Read the model definition and answer for the solid it produces. Units are mm, in the model's axes. Face numbers are marked on the shaded views. A direction names the side the tool comes from. Coordinates: 2 decimals unless noted, no trailing zeros. Order: outer loops, then holes, each group sorted by start corner. A loop starts at its lowest first (then second) coordinate and runs counter-clockwise, first axis right, second up. Notation, with made-up numbers: M 71.5,38 L 120.5,38 A16 cw 120.5,56 Z; hole C -2,-26 d6. An arc over 180 degrees is marked long. Use a Markdown table: item, result. Add a question column.
1) Find the intervals of material crossed by probe 1 along X at (y, z) = (49, 1.75); probe 2 along Y at (x, z) = (2.5, 2); probe 3 along X at (y, z) = (73, 3), in increasing order. Write a range as [from, to].
2) Each of these flat-tipped pins is pushed along its axis until it touches: pin 1 Ø7.5 at (x, y) = (58, 50) entering from -Z; pin 2 Ø1 at (y, z) = (57, 1) entering from -X; pin 3 Ø1.2 at (x, z) = (1, 0.5) entering from -Y; pin 4 Ø2.5 at (x, y) = (-59.98, 54.01) entering from +Z. Where does it stop, or does it pass through?
3) Find section A-A on z = 3.75. Write down the section's boundary in (x, y), plus the area to 3 significant figures.
4) The mould has two halves that part along X. Classify the marked faces 4, 5, 6 and 7: released by +X, released by -X, zero draft, split by the parting line, or undercut.
5) For the marked faces 1, 2 and 3, determine the directions among +Z, -Z, +X, -X, +Y, -Y from which every point of the face is accessible in a straight line to the end or side of a thin tool.
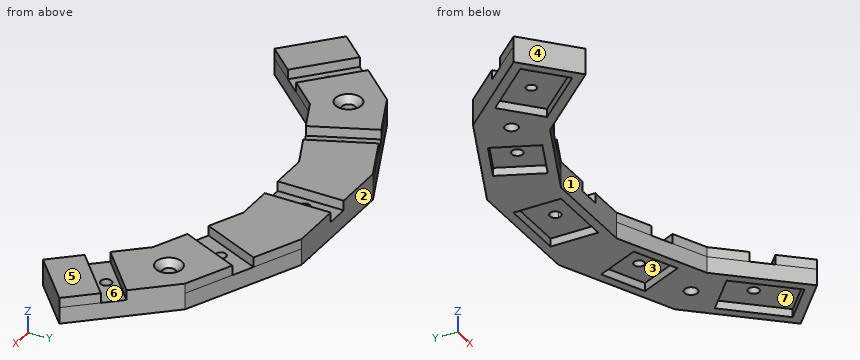
from build123d import *

# Parameters (mm, degrees)
F1_DEPTH       = 5
F3_DEPTH       = 3
F6_D           = 4
F6_CSINK_D     = 8
F6_CSINK_ANGLE = 90
F4_R           = 1.5456356791
F4_R_2         = 1.6934971507
F4_R_3         = 1.5922062155
F4_R_4         = 1.6882702818
F7_DEPTH       = 11.1
F9_DEPTH       = 2.5
F10_R          = 1.4984626167
F11_DEPTH      = 1
F12_R          = 1.6745754143
F13_DEPTH      = 1
F14_W          = 7
F14_H          = 20.1999992132
F14_R          = 1.6202134685
F15_DEPTH      = 1
F16_R          = 1.6358408112
F17_DEPTH      = 1
F18_R          = 1.6662774654
F19_DEPTH      = 1


with BuildPart() as f1:
    # F0 (on Top) → F1 (new body)
    with BuildSketch(Plane.XY):
        Polygon((-42.3623017311, 58.3067062123), (-14.9844143682, 70.4961270094), (14.9844143682, 70.4961270094), (42.3623017311, 58.3067062123), (62.4153622753, 36.0355262112), (77.4268871653, 49.5519639332), (54.5008190929, 75.0139420503), (19.2780567467, 90.6961262226), (-19.2780567467, 90.6961262226), (-54.5008190929, 75.0139420503), (-77.4268871653, 49.5519639332), (-62.4153622753, 36.0355262112), align=None)
    extrude(amount=F1_DEPTH)

    # F2 (on face) → F3 (join)
    with BuildSketch(Plane.XY.offset(5)):
        Polygon((19.2780567467, 90.6961262226), (3.5, 90.6961262226), (3.5, 70.4961270094), (14.9844143682, 70.4961270094), (25.532006503, 65.80003643), (33.7641456248, 84.2464955399), align=None)
        Polygon((-3.5, 70.4961270094), (-3.5, 90.6961262226), (-19.2780567467, 90.6961262226), (-33.7641456248, 84.2464955399), (-25.532006503, 65.80003643), (-14.9844143682, 70.4961270094), align=None)
        Polygon((54.5008190929, 75.0139420503), (40.1589641997, 81.3993472492), (31.9268219148, 62.9528811714), (42.3623017311, 58.3067062123), (50.1289961086, 49.6809182377), (65.1640507517, 63.1712235215), align=None)
        Polygon((77.4268871653, 49.5519639332), (69.8479569532, 57.9692186757), (54.8129021735, 44.4789135438), (62.4153622753, 36.0355262112), align=None)
        Polygon((-31.9268219148, 62.9528811714), (-40.1589641997, 81.3993472492), (-54.5008190929, 75.0139420503), (-65.1640507517, 63.1712235215), (-50.1289961086, 49.6809182377), (-42.3623017311, 58.3067062123), align=None)
        Polygon((-54.8129021735, 44.4789135438), (-69.8479569532, 57.9692186757), (-77.4268871653, 49.5519639332), (-62.4153622753, 36.0355262112), align=None)
    extrude(amount=F3_DEPTH)

    # F6 (through all)
    with Locations(Plane.XY.offset(8)):
        with Locations((-48.431560412, 66.6603241313), (48.431560412, 66.6603241313)):
            CounterSinkHole(F6_D / 2, F6_CSINK_D / 2, counter_sink_angle=F6_CSINK_ANGLE)

    # F4 (on face) → F7 (cut)
    with BuildSketch(Plane.XY.offset(5)):
        with BuildLine():
            ThreePointArc((1.6936241921, 80.7094499469), (1.197573151, 81.9070230979), (0, 82.403074139))
            Line((0, 82.403074139), (0, 79.0158257547))
            ThreePointArc((0, 79.0158257547), (1.197573151, 79.5118767958), (1.6936241921, 80.7094499469))
        make_face()
        with BuildLine():
            Line((0, 79.0158257547), (0, 82.403074139))
            ThreePointArc((0, 82.403074139), (-1.6936241921, 80.7094499469), (0, 79.0158257547))
        make_face()
        with Locations((-59.9788100952, 54.0051631818)):
            Circle(F4_R)
        with Locations((-32.8274907359, 73.7317513878)):
            Circle(F4_R_2)
        with Locations((32.8274907359, 73.7317513878)):
            Circle(F4_R_3)
        with Locations((59.9788100952, 54.0051631818)):
            Circle(F4_R_4)
    extrude(amount=-F7_DEPTH, mode=Mode.SUBTRACT)

    # F8 (on face) → F9 (cut)
    with BuildSketch(Plane(origin=(0, 0, 0), x_dir=(1, 0, 0), z_dir=(0, 0, -1))):
        Polygon((62.6226022883, -39.9899012252), (48.4079691697, -55.7768506604), (59.2578790327, -65.5461533813), (73.4725121513, -49.7592039462), align=None)
        Polygon((23.2004942383, -69.9030770993), (29.1388467156, -83.2408351397), (42.3623017311, -77.3533736479), (36.4239492538, -64.0156156075), align=None)
        Polygon((-10.046819225, -73.2961297035), (-10.046819225, -87.8961235285), (10.046819225, -87.8961235285), (10.046819225, -73.2961297035), (0, -73.2961297035), align=None)
        Polygon((-23.2004942383, -69.9030770993), (-36.4239492538, -64.0156156075), (-42.3623017311, -77.3533736479), (-29.1388467156, -83.2408351397), align=None)
        Polygon((-48.4079691697, -55.7768506604), (-62.6226022883, -39.9899012252), (-73.4725121513, -49.7592039462), (-59.2578790327, -65.5461533813), align=None)
    extrude(amount=-F9_DEPTH, mode=Mode.SUBTRACT)


with BuildPart() as f11:
    # F10 (on face) → F11 (new body)
    with BuildSketch(Plane.XY.offset(5)):
        Polygon((-50.1289961086, 49.6809182377), (-65.1640507517, 63.1712235215), (-69.8479569532, 57.9692186757), (-54.8129021735, 44.4789135438), align=None)
        with Locations((-59.9788100952, 54.0051631818)):
            Circle(F10_R, mode=Mode.SUBTRACT)
    extrude(amount=F11_DEPTH)


with BuildPart() as f13:
    # F12 (on face) → F13 (new body)
    with BuildSketch(Plane.XY.offset(5)):
        Polygon((-25.532006503, 65.80003643), (-33.7641487432, 84.2465025277), (-40.1589641997, 81.3993472492), (-31.9268219148, 62.9528811714), align=None)
        with Locations((-32.8274907359, 73.7317513878)):
            Circle(F12_R, mode=Mode.SUBTRACT)
    extrude(amount=F13_DEPTH)


with BuildPart() as f15:
    # F14 (on face) → F15 (new body)
    with BuildSketch(Plane.XY.offset(5)):
        with Locations((0, 80.596126616)):
            Rectangle(F14_W, F14_H)
        with Locations((0, 80.7094499469)):
            Circle(F14_R, mode=Mode.SUBTRACT)
    extrude(amount=F15_DEPTH)


with BuildPart() as f17:
    # F16 (on face) → F17 (new body)
    with BuildSketch(Plane.XY.offset(5)):
        Polygon((40.1589641997, 81.3993472492), (33.7641487432, 84.2465025277), (25.532006503, 65.80003643), (31.9268219148, 62.9528811714), align=None)
        with Locations((32.8274907359, 73.7317513878)):
            Circle(F16_R, mode=Mode.SUBTRACT)
    extrude(amount=F17_DEPTH)


with BuildPart() as f19:
    # F18 (on face) → F19 (new body)
    with BuildSketch(Plane.XY.offset(5)):
        Polygon((69.8479569532, 57.9692186757), (65.1640507517, 63.1712235215), (50.1289961086, 49.6809182377), (54.8129021735, 44.4789135438), align=None)
        with Locations((59.9788100952, 54.0051631818)):
            Circle(F18_R, mode=Mode.SUBTRACT)
    extrude(amount=F19_DEPTH)


solid = f1.part
Check result:
| question | item | result |
|---|---|---|
| 1 | probe 1 | x = [-76.81, -72.63], [-54.51, -50.74], [50.74, 54.51], [72.63, 76.81] |
| 1 | probe 2 | y = [70.5, 73.3], [87.9, 90.7] |
| 1 | probe 3 | x = [-56.31, -34.35], [-31.3, 31.41], [34.24, 56.31] |
| 2 | pin 1 | stops at z = 0 |
| 2 | pin 2 | stops at x = -71.17 |
| 2 | pin 3 | stops at y = 70.5 |
| 2 | pin 4 | passes through |
| 3 | outline | M -77.43,49.55 L -62.42,36.04 L -42.36,58.31 L -14.98,70.5 L 14.98,70.5 L 42.36,58.31 L 62.42,36.04 L 77.43,49.55 L 54.5,75.01 L 19.28,90.7 L -19.28,90.7 L -54.5,75.01 Z; hole C -59.98,54.01 d3.09; hole C -48.43,66.66 d4; hole C -32.83,73.73 d3.39; hole C 0,80.71 d3.39; hole C 32.83,73.73 d3.18; hole C 48.43,66.66 d4; hole C 59.98,54.01 d3.38 |
| 3 | area | 3,310 mm2 |
| 4 | face 4 | released by -X |
| 4 | face 5 | zero draft |
| 4 | face 6 | undercut |
| 4 | face 7 | undercut |
| 5 | face 1 | +Z, -Z, -Y |
| 5 | face 2 | +Z, -Z, +X, -X, +Y |
| 5 | face 3 | -Z |
